Check sheet for the drawn part. Datum: minimum x, y, z corner. Units: mm. A direction names the side the tool comes from. Give positions to 0.01 mm unless a question says otherwise; leave off trailing zeros. Loops run counter-clockwise (first coordinate to the right, second up) from the corner with the lowest first, then second, coordinate; pieces in that order, holes last.
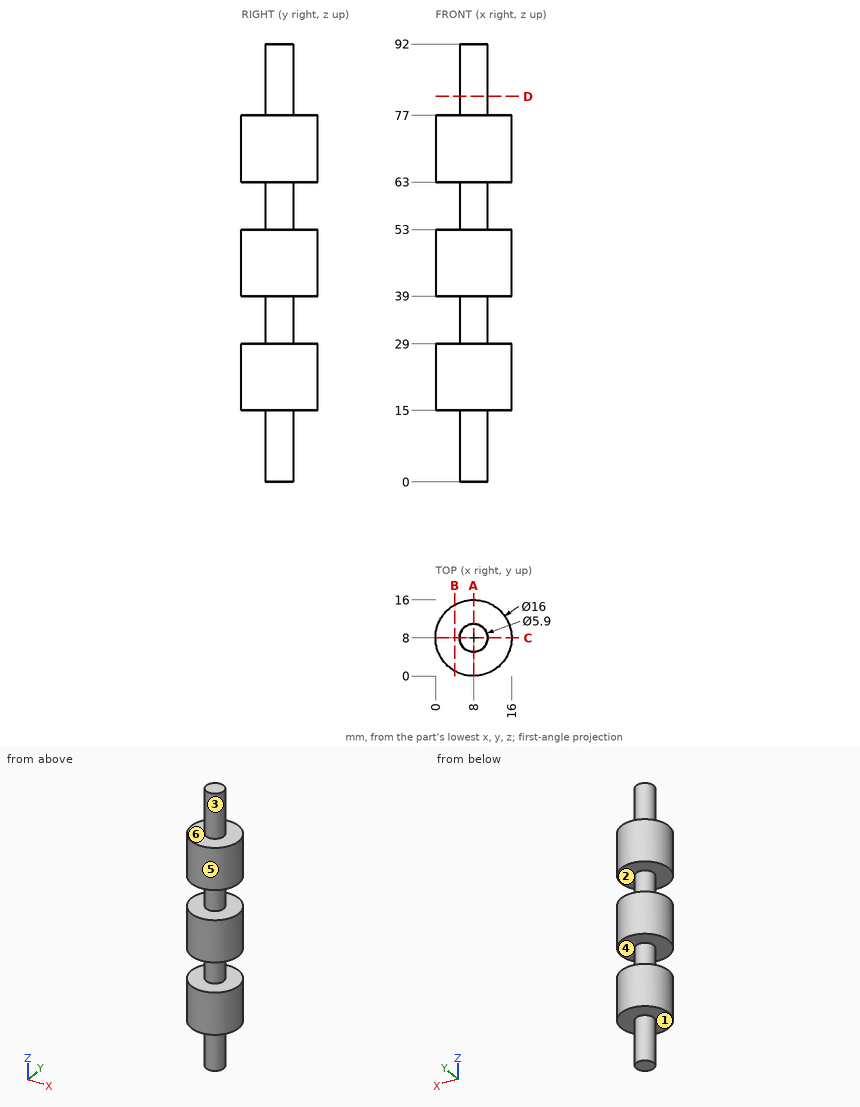
(1) Release check for a two-part mould opening along Z. For the marked faces 4, 5 and 6 record: pulls with the +Z half, pulls with the -Z half, needs draft (parallel to the pull), parting line crosses it, or undercut.
(2) Access from +Z, -Z, +X, -X, +Y, -Y to the whole of each face (thin tool, end or side, straight path). Record for the marked faces 1, 2 and 3.
(3) Section check B-B on x = 4. Record the boundary of the cut face in (y, z).
(4) Section check A-A on x = 8. Record the boundary of the cut face in (y, z).
(5) Gauge pin test, flat ends, axial feed: pin 1 Ø1 at (x, y) = (13.5, 12.5) entering from -Z; pin 2 Ø3 at (x, y) = (4, 11) entering from +Z; pin 3 Ø1 at (y, z) = (3.5, 68.5) entering from +X. Record the tip position at first contact, or that the pin passes through.
(6) Material ranges on line 1 (Z direction, x = 1.5, y = 11.25); line 2 (Y direction, x = 10.5, z = 73.5); line 3 (Y direction, x = 1.25, z = 76), recorded low to high.
(7) Section check D-D on z = 81. Record the boundary of the cut face in (x, y), plus the area to 3 significant figures.
Computed values:
1. face 4: undercut
1. face 5: needs draft
1. face 6: pulls with the +Z half
2. face 1: -Z
2. face 2: none
2. face 3: +Z
3. outline: (1.07, 15) - (14.93, 15) - (14.93, 29) - (1.07, 29) - close; (1.07, 39) - (14.93, 39) - (14.93, 53) - (1.07, 53) - close; (1.07, 63) - (14.93, 63) - (14.93, 77) - (1.07, 77) - close
4. outline: (0, 15) - (5.05, 15) - (5.05, 0) - (10.95, 0) - (10.95, 15) - (16, 15) - (16, 29) - (10.95, 29) - (10.95, 39) - (16, 39) - (16, 53) - (10.95, 53) - (10.95, 63) - (16, 63) - (16, 77) - (10.95, 77) - (10.95, 92) - (5.05, 92) - (5.05, 77) - (0, 77) - (0, 63) - (5.05, 63) - (5.05, 53) - (0, 53) - (0, 39) - (5.05, 39) - (5.05, 29) - (0, 29) - close
5. pin 1: stops at z = 15
5. pin 2: stops at z = 77
5. pin 3: stops at x = 14.93
6. line 1: z = 15 to 29, 39 to 53, 63 to 77
6. line 2: y = 0.4 to 15.6
6. line 3: y = 3.71 to 12.29
7. outline: circle Ø5.9 at (8, 8)
7. area: 27.3 mm2
